Check sheet for the modelled part. Datum: model origin and axes. Units: mm. A direction names the side the tool comes from. Give positions to 0.01 mm unless a question says otherwise; leave off trailing zeros. Loops run counter-clockwise (first coordinate to the right, second up) from the corner with the lowest first, then second, coordinate; pieces in that order, holes last. Notation, with made-up numbers: (85.5, 34) - (119.5, 34) arc R22 ccw to (119.5, 62) - close; hole circle Ø11 at (31.25, 26.25). An arc over 180 degrees is marked (long way). Answer in a Markdown table with one row per item. Add a question column.
(1) Draft check along X on faces 1 (the face through (-40.72, 113.64, 38.62)), 2 (the face through (25, 109, 20)), 3 (the face through (-57.15, 33.01, 38.62)). Enter one of: released by +X, released by -X, zero draft, split by the parting line, or undercut.
(2) Sectioned sample at A-A on x = 0. Enter the section's corners in (y, z) (3 decimals), then the cut area to 3 significant figures.
(3) Sectioned sample at C-C on y = 45. Enter the section's corners in (x, z) (3 decimals), then the cut area to 3 significant figures.
(4) Sectioned sample at B-B on z = 0. Enter the section's corners in (x, y) (3 decimals), then the cut area to 3 significant figures.
(5) Sectioned sample at D-D on x = -40. State how many separate pieces and enclosed holes the cut face has, then the cut area to 3 significant figures.
(6) Thickness scan on L1, parallel to Y at x = -40, z = 38.5 (1 decimal); L2, parallel to Z at x = 9.5, y = 68.5; L3, parallel to X at y = 52, z = 21 (3 decimals). Record the ranges inside material, lowest first.
(7) Go/stop test with flat-tipped pins: P1, Ø1.5, axis at x = -6, y = 96, coming from the -Z side; P2, Ø17.5, axis at x = 40, y = 171.375, coming from the -Z side; P3, Ø5, axis at x = 17.5, y = 181.5, coming from the -Z side. Record where each tip stops, or that it passes through.
(8) Set-up check for faces 4 (the face through (-21.825, 109, 24)), 5 (the face through (-17.669, 183.883, -11.265)), 6 (the face through (17, 38.1, 9.2)): record each of +Z, -Z, +X, -X, +Y, -Y from which the full face is reachable in a straight line by a thin tool's end or side.
from build123d import *

# Parameters (mm, degrees)
BOSS_EXTRUDE1_START   = -3.175
BOSS_EXTRUDE1_DEPTH   = 3.175
BOSS_EXTRUDE9_START   = -153.2
BOSS_EXTRUDE9_DEPTH   = 153.2
BOSS_EXTRUDE5_START   = 3.175
BOSS_EXTRUDE5_DEPTH   = 3.175
SKETCH18_W            = 120
SKETCH18_H            = 156.375
BOSS_EXTRUDE10_DEPTH  = 6.35
FILLET1_R             = 10
M10_CLEARANCE_HOLE2_D = 11


with BuildPart() as part:
    # Sketch12 → Revolve1 (revolve)
    with BuildSketch(Plane.XY, mode=Mode.PRIVATE) as revolve1_sk:
        Polygon((-25.399999994, 0), (-25.399999994, 203.2), (-20.955, 203.2), (-20.955, 165.1), (-19.177, 165.1), (-19.177, 38.1), (-20.955, 38.1), (-20.955, 0), align=None)
    revolve(revolve1_sk.sketch.rotate(Axis((0, 0, 0), (0, 1, 0)), 270), axis=Axis((0, 0, 0), (0, 1, 0)))

    # Sketch14 → Boss-Extrude1 (add)
    with BuildSketch(Plane(origin=(0, 30, 0), x_dir=(-1, 0, 0), z_dir=(0, -1, 0)).offset(BOSS_EXTRUDE1_START)):
        with BuildLine():
            Line((-21.825, -12.993435831), (-21.825, -35.399999994))
            Line((-21.825, -35.399999994), (21.825, -35.399999994))
            Line((21.825, -35.399999994), (21.825, -12.993435831))
            ThreePointArc((21.825, -12.993435831), (0, -25.399999994), (-21.825, -12.993435831))
        make_face()
    extrude(amount=BOSS_EXTRUDE1_DEPTH)

    # Sketch14<4> → Boss-Extrude9 (add)
    with BuildSketch(Plane(origin=(0, 30, 0), x_dir=(-1, 0, 0), z_dir=(0, -1, 0)).offset(BOSS_EXTRUDE9_START)):
        with BuildLine():
            Line((-25, -4.489988829), (-25, -35.399999994))
            Line((-25, -35.399999994), (-21.825, -35.399999994))
            Line((-21.825, -35.399999994), (-21.825, -12.993435831))
            ThreePointArc((-21.825, -12.993435831), (-23.79542622, -8.884688554), (-25, -4.489988829))
        make_face()
        with BuildLine():
            Line((21.825, -12.993435831), (21.825, -35.399999994))
            Line((21.825, -35.399999994), (25, -35.399999994))
            Line((25, -35.399999994), (25, -4.489988829))
            ThreePointArc((25, -4.489988829), (23.79542622, -8.884688554), (21.825, -12.993435831))
        make_face()
    extrude(amount=BOSS_EXTRUDE9_DEPTH)

    # Sketch17 → Boss-Extrude5 (add)
    with BuildSketch(Plane(origin=(0, 183.2, 0), x_dir=(1, 0, 0), z_dir=(0, 1, 0)).offset(BOSS_EXTRUDE5_START)):
        with BuildLine():
            Line((25, -35.399999994), (25, -4.489988829))
            ThreePointArc((25, -4.489988829), (0, -25.399999994), (-25, -4.489988829))
            Line((-25, -4.489988829), (-25, -35.399999994))
            Line((-25, -35.399999994), (25, -35.399999994))
        make_face()
    extrude(amount=-BOSS_EXTRUDE5_DEPTH)

    # Sketch18 → Boss-Extrude10 (add)
    with BuildSketch(Plane.XY.offset(35.399999994)):
        with Locations((0, 108.1875)):
            Rectangle(SKETCH18_W, SKETCH18_H)
    extrude(amount=BOSS_EXTRUDE10_DEPTH)

    # Fillet1
    fillet1_edges = [part.edges().sort_by_distance(p)[0] for p in [
        (-60, 186.375, 38.574999994),
        (-60, 30, 38.574999994),
        (60, 30, 38.574999994),
        (60, 186.375, 38.574999994),
    ]]
    fillet(fillet1_edges, radius=FILLET1_R)

    # M10 Clearance Hole2 (through all)
    with Locations(Plane(origin=(-40, 45, 35.399999994), x_dir=(-1, 0, 0), z_dir=(0, 0, -1))):
        with Locations((0, 0), (0, 63.1875), (0, 126.375), (-80, 126.375), (-80, 63.1875), (-80, 0)):
            Hole(M10_CLEARANCE_HOLE2_D / 2)


solid = part.part
Reply:
| question | item | result |
|---|---|---|
| 1 | face 1 | undercut |
| 1 | face 2 | released by +X |
| 1 | face 3 | released by -X |
| 2 | outline | (0, -25.4) - (203.2, -25.4) - (203.2, -20.955) - (165.1, -20.955) - (165.1, -19.177) - (38.1, -19.177) - (38.1, -20.955) - (0, -20.955) - close; (0, 20.955) - (38.1, 20.955) - (38.1, 19.177) - (165.1, 19.177) - (165.1, 20.955) - (203.2, 20.955) - (203.2, 25.4) - (186.375, 25.4) - (186.375, 41.75) - (30, 41.75) - (30, 25.4) - (0, 25.4) - close; hole (33.175, 25.4) - (183.2, 25.4) - (183.2, 35.4) - (33.175, 35.4) - close |
| 2 | area | 3,310 mm^2 |
| 3 | outline | (-60, 35.4) - (-45.5, 35.4) - (-45.5, 41.75) - (-60, 41.75) - close; (-34.5, 35.4) - (-25, 35.4) - (-25, 4.49) arc R25.4 ccw (long way) to (25, 4.49) - (25, 35.4) - (34.5, 35.4) - (34.5, 41.75) - (-34.5, 41.75) - close; (45.5, 35.4) - (60, 35.4) - (60, 41.75) - (45.5, 41.75) - close; hole (-21.825, 12.993) arc R25.4 cw to (21.825, 12.993) - (21.825, 35.4) - (-21.825, 35.4) - close; hole circle Ø38.354 at (0, 0) |
| 3 | area | 1,660 mm^2 |
| 4 | outline | (-25.4, 0) - (-20.955, 0) - (-20.955, 38.1) - (-19.177, 38.1) - (-19.177, 165.1) - (-20.955, 165.1) - (-20.955, 203.2) - (-25.4, 203.2) - close; (19.177, 38.1) - (20.955, 38.1) - (20.955, 0) - (25.4, 0) - (25.4, 203.2) - (20.955, 203.2) - (20.955, 165.1) - (19.177, 165.1) - close |
| 4 | area | 2,260 mm^2 |
| 5 | separate pieces | 4 |
| 5 | enclosed holes | 0 |
| 5 | area | 783 mm^2 |
| 6 | L1 | 30 to 39.5, 50.5 to 102.7, 113.7 to 165.9, 176.9 to 186.4 |
| 6 | L2 | -23.56 to -16.66, 16.66 to 23.56, 35.4 to 41.75 |
| 6 | L3 | -25 to -21.825, -14.288 to 14.288, 21.825 to 25 |
| 7 | P1 | z = -24.85 |
| 7 | P2 | z = 35.4 |
| 7 | P3 | z = -20.5 |
| 8 | face 4 | none |
| 8 | face 5 | +Y |
| 8 | face 6 | -Y |
